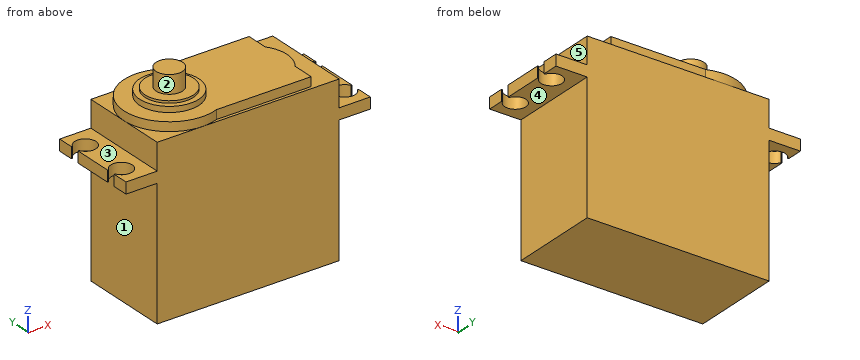
```python
from build123d import *

# Parameters (mm, degrees)
SKIZZE1_W                       = 40.2
SKIZZE1_H                       = 36.8
AUFSATZ_LINEAR_AUSTRAGEN1_DEPTH = 20
AUFSATZ_LINEAR_AUSTRAGEN2_DEPTH = 2
SKIZZE3_R                       = 6.535
AUFSATZ_LINEAR_AUSTRAGEN3_DEPTH = 1.25
SKIZZE4_R                       = 5.35
AUFSATZ_LINEAR_AUSTRAGEN4_DEPTH = 0.5
SKIZZE5_R                       = 2.925
AUFSATZ_LINEAR_AUSTRAGEN5_DEPTH = 4
AUFSATZ_LINEAR_AUSTRAGEN6_DEPTH = 2.46


with BuildPart() as part:
    # Skizze1 → Aufsatz-Linear austragen1 (new body)
    with BuildSketch(Plane(origin=(0, 0, 0), x_dir=(1, 0, 0), z_dir=(0, 1, 0))):
        Rectangle(SKIZZE1_W, SKIZZE1_H)
    extrude(amount=AUFSATZ_LINEAR_AUSTRAGEN1_DEPTH)

    # Skizze2 → Aufsatz-Linear austragen2 (add)
    with BuildSketch(Plane.XY.offset(18.4)):
        with BuildLine():
            Line((-6.553522875, 19.35), (14.4, 19.35))
            Line((14.4, 19.35), (14.4, 14.5))
            ThreePointArc((14.4, 14.5), (15.9, 10), (14.4, 5.5))
            Line((14.4, 5.5), (14.4, 0.65))
            Line((14.4, 0.65), (-6.553522875, 0.65))
            ThreePointArc((-6.553522875, 0.65), (-20.1, 10), (-6.553522875, 19.35))
        make_face()
    extrude(amount=AUFSATZ_LINEAR_AUSTRAGEN2_DEPTH)

    # Skizze3 → Aufsatz-Linear austragen3 (add)
    with BuildSketch(Plane.XY.offset(20.4)):
        with Locations((-10.1, 10)):
            Circle(SKIZZE3_R)
    extrude(amount=AUFSATZ_LINEAR_AUSTRAGEN3_DEPTH)

    # Skizze4 → Aufsatz-Linear austragen4 (add)
    with BuildSketch(Plane.XY.offset(21.65)):
        with Locations((-10.1, 10)):
            Circle(SKIZZE4_R)
    extrude(amount=AUFSATZ_LINEAR_AUSTRAGEN4_DEPTH)

    # Skizze5 → Aufsatz-Linear austragen5 (add)
    with BuildSketch(Plane.XY.offset(22.15)):
        with Locations((-10.1, 10)):
            Circle(SKIZZE5_R)
    extrude(amount=AUFSATZ_LINEAR_AUSTRAGEN5_DEPTH)

    # Skizze6 → Aufsatz-Linear austragen6 (add)
    with BuildSketch(Plane(origin=(0, 0, 10.1), x_dir=(-1, 0, 0), z_dir=(0, 0, -1))):
        with BuildLine():
            Line((20.1, 20), (20.1, 0))
            Line((20.1, 0), (27, 0))
            Line((27, 0), (27, 3.55))
            Line((27, 3.55), (26.776617032, 3.55))
            ThreePointArc((26.776617032, 3.55), (22.3, 4.55), (26.776617032, 5.55))
            Line((26.776617032, 5.55), (27, 5.55))
            Line((27, 5.55), (27, 14.45))
            Line((27, 14.45), (26.776617032, 14.45))
            ThreePointArc((26.776617032, 14.45), (22.3, 15.45), (26.776617032, 16.45))
            Line((26.776617032, 16.45), (27, 16.45))
            Line((27, 16.45), (27, 20))
            Line((27, 20), (20.1, 20))
        make_face()
        with BuildLine():
            Line((-27, 3.55), (-27, 0))
            Line((-27, 0), (-20.1, 0))
            Line((-20.1, 0), (-20.1, 20))
            Line((-20.1, 20), (-27, 20))
            Line((-27, 20), (-27, 16.45))
            Line((-27, 16.45), (-26.776617032, 16.45))
            ThreePointArc((-26.776617032, 16.45), (-22.3, 15.45), (-26.776617032, 14.45))
            Line((-26.776617032, 14.45), (-27, 14.45))
            Line((-27, 14.45), (-27, 5.55))
            Line((-27, 5.55), (-26.776617032, 5.55))
            ThreePointArc((-26.776617032, 5.55), (-22.3, 4.55), (-26.776617032, 3.55))
            Line((-26.776617032, 3.55), (-27, 3.55))
        make_face()
    extrude(amount=-AUFSATZ_LINEAR_AUSTRAGEN6_DEPTH)


solid = part.part
```
Can you work these out from the model? Positions are in its coordinate system, mm. Face numbers are marked on the shaded views. A direction names the side the tool comes from. Coordinates: 2 decimals unless noted, no trailing zeros. Write each loop counter-clockwise with the first axis right and the second up, starting at its lowest first coordinate (ties: lowest second). Pieces come first, ordered by that corner, then holes. Notation, with made-up numbers: M 59,84.25 L 98,84.25 A13 ccw 98,92.25 Z; hole C 88,10 d10. An arc over 180 degrees is marked long. Answer as CSV lines item,"result".
Item 1: Please list where these lines run through material, in increasing order: line 1 along Y through (x, z) = (-24.65, 11.05); line 2 along X through (y, z) = (5.5, -10); line 3 along Z through (x, y) = (17.5, 1.25).
Geometry results:
line 1,"y = 0 to 2.2, 6.9 to 13.1, 17.8 to 20"
line 2,"x = -20.1 to 20.1"
line 3,"z = -18.4 to 18.4"
Item 2: On a 3-axis mill with a long thin cutter (end or side, diameter ignored), from which of +Z, -Z, +X, -X, +Y, -Y can I reach the whole of each face in a straight line? I mean the marked faces 1, 2, 3, 4 and 5. Say none if no direction works.
Geometry results:
face 1,"-Z, -X, +Y, -Y"
face 2,"+Z"
face 3,"+Z, -X, +Y, -Y"
face 4,"-Z, +X, +Y, -Y"
face 5,"+Z, +X, +Y, -Y"
Item 3: Imagine slicing it at B-B on x = -0.5. List the corners of the cut face in (y, z) for me, plus the area to 3 significant figures.
Geometry results:
outline,"M 0,-18.4 L 20,-18.4 L 20,18.4 L 19.35,18.4 L 19.35,20.4 L 0.65,20.4 L 0.65,18.4 L 0,18.4 Z"
area,"773 mm2"
Item 4: Imagine slicing it at D-D on z = 14. List the corners of the cut face in (x, y) for me, plus the area to 3 significant figures.
Geometry results:
outline,"M -20.1,0 L 20.1,0 L 20.1,20 L -20.1,20 Z"
area,"804 mm2"
Item 5: Imagine slicing it at C-C on y = 12. List the corners of the cut face in (x, z) for me.
Geometry results:
outline,"M -27,10.1 L -20.1,10.1 L -20.1,-18.4 L 20.1,-18.4 L 20.1,10.1 L 27,10.1 L 27,12.56 L 20.1,12.56 L 20.1,18.4 L 15.63,18.4 L 15.63,20.4 L -3.88,20.4 L -3.88,21.65 L -5.14,21.65 L -5.14,22.15 L -7.97,22.15 L -7.97,26.15 L -12.23,26.15 L -12.23,22.15 L -15.06,22.15 L -15.06,21.65 L -16.32,21.65 L -16.32,20.4 L -19.9,20.4 L -19.9,18.4 L -20.1,18.4 L -20.1,12.56 L -27,12.56 Z"
Item 6: Imagine slicing it at A-A on x = -24.65. List the corners of the cut face in (y, z) for me, plus the area to 3 significant figures.
Geometry results:
outline,"M 0,10.1 L 2.2,10.1 L 2.2,12.56 L 0,12.56 Z; M 6.9,10.1 L 13.1,10.1 L 13.1,12.56 L 6.9,12.56 Z; M 17.8,10.1 L 20,10.1 L 20,12.56 L 17.8,12.56 Z"
area,"26.1 mm2"
Item 7: I'm going to push flat-ended pins straight in: P1, Ø4, axis at y = 3, z = -6, coming from the -X side; P2, Ø6.5, axis at y = 12, z = 14.5, coming from the -X side; P3, Ø3, axis at y = 4, z = 21.5, coming from the +X side; P4, Ø4, axis at x = 1.5, y = 13.5, coming from the +Z side. Where does each tip first touch, or does it pass through?
Geometry results:
P1,"stops at x = -20.1"
P2,"stops at x = -27"
P3,"stops at x = 14.4"
P4,"stops at z = 20.4"
